from build123d import *

# Parameters (mm, degrees)
SKETCH1_W           = 21
SKETCH1_H           = 15
BOSS_EXTRUDE1_DEPTH = 3
SKETCH2_W           = 4
SKETCH2_H           = 15
BOSS_EXTRUDE2_DEPTH = 14.5
SKETCH3_W           = 4
SKETCH3_H           = 7
SKETCH3_W_2         = 4.5
SKETCH3_H_2         = 4
BOSS_EXTRUDE3_DEPTH = 3.5
FILLET1_R           = 1
FILLET2_R           = 3
FILLET3_R           = 5
SKETCH4_W           = 8
SKETCH4_H           = 10
SKETCH4_R           = 1.75
BOSS_EXTRUDE4_DEPTH = 3
FILLET4_R           = 5
FILLET5_R           = 2
SKETCH7_W           = 8
SKETCH7_H           = 4
BOSS_EXTRUDE5_DEPTH = 10
SKETCH8_W           = 4
SKETCH8_H           = 3
BOSS_EXTRUDE6_DEPTH = 8
SKETCH9_R           = 4.5
CUT_EXTRUDE1_DEPTH  = 5
BOSS_EXTRUDE7_DEPTH = 6.5
SKETCH11_R          = 1.75
SKETCH11_W          = 2
SKETCH11_H          = 7.704965023
BOSS_EXTRUDE8_DEPTH = 3
FILLET6_R           = 4
FILLET7_START       = -17.5
FILLET7_DEPTH       = 3
FILLET7_START_2     = -14.5
FILLET7_2_DEPTH     = 3.464101615
FILLET7_START_3     = -6.795034977
FILLET7_3_DEPTH     = 4.795034977
FILLET8_R           = 3
FILLET9_R           = 3
FILLET10_R          = 1.5


with BuildPart() as part:
    # Sketch1 → Boss-Extrude1 (new body)
    with BuildSketch(Plane.XY):
        Rectangle(SKETCH1_W, SKETCH1_H)
    extrude(amount=-BOSS_EXTRUDE1_DEPTH)

    # Sketch2 → Boss-Extrude2 (add)
    with BuildSketch(Plane(origin=(0, 0, -3), x_dir=(-1, 0, 0), z_dir=(0, 0, -1))):
        with Locations((8.5, 0)):
            Rectangle(SKETCH2_W, SKETCH2_H)
        with Locations((-8.5, 0)):
            Rectangle(SKETCH2_W, SKETCH2_H)
    extrude(amount=BOSS_EXTRUDE2_DEPTH)

    # Sketch3 → Boss-Extrude3 (add)
    with BuildSketch(Plane(origin=(0, 0, -17.5), x_dir=(-1, 0, 0), z_dir=(0, 0, -1))):
        with Locations((8.5, 11)):
            Rectangle(SKETCH3_W, SKETCH3_H)
        with Locations((4.25, 12.5)):
            Rectangle(SKETCH3_W_2, SKETCH3_H_2)
    extrude(amount=-BOSS_EXTRUDE3_DEPTH)

    # Fillet1
    fillet1_edges = [part.edges().sort_by_distance(p)[0] for p in [
        (-6.25, 14.5, -14),
        (-2, 14.5, -15.75),
    ]]
    fillet(fillet1_edges, radius=FILLET1_R)

    # Fillet2
    # the kernel refuses this fillet: 3 mm, written as the material it takes off along each edge
    with BuildSketch(Plane(origin=(-5, 14.5, -17), x_dir=(0, 0, 1), z_dir=(-1, 0, 0))) as fillet2_piece_1:
        with BuildLine():
            CenterArc((2, -1), 1, 0, 90)
            Line((3, -1), (3, 0))
            Line((3, 0), (2, 0))
        make_face()
    revolve(axis=Axis((-5, 14.5, -17), (0, 1, 0)), revolution_arc=90, mode=Mode.SUBTRACT)
    with BuildSketch(Plane(origin=(-2, 14.5, -14), x_dir=(0, 0, -1), z_dir=(0, -1, 0))) as fillet2_piece_2:
        with BuildLine():
            CenterArc((FILLET2_R, -FILLET2_R), FILLET2_R, 90, 90)
            Line((0, -FILLET2_R), (0, 0))
            Line((0, 0), (FILLET2_R, 0))
        make_face()
    extrude(amount=11.5, mode=Mode.SUBTRACT)

    # Fillet3
    # the kernel refuses this fillet: 5 mm, written as the material it adds along each edge
    with BuildSketch(Plane(origin=(-10.5, 7.5, -14), x_dir=(0, 1, 0), z_dir=(1, 0, 0))) as fillet3_piece_1:
        with BuildLine():
            CenterArc((FILLET3_R, FILLET3_R), FILLET3_R, 180, 90)
            Line((0, FILLET3_R), (0, 0))
            Line((0, 0), (FILLET3_R, 0))
        make_face()
    extrude(amount=4)

    # Sketch4 → Boss-Extrude4 (add)
    with BuildSketch(Plane(origin=(0, 0, -17.5), x_dir=(-1, 0, 0), z_dir=(0, 0, -1))):
        with Locations((14.5, 0.098378943)):
            Rectangle(SKETCH4_W, SKETCH4_H)
        with Locations((14.5, 0.098378943)):
            Circle(SKETCH4_R, mode=Mode.SUBTRACT)
    extrude(amount=-BOSS_EXTRUDE4_DEPTH)

    # Fillet4
    # the kernel refuses this fillet: 5 mm, written as the material it adds along each edge
    with BuildSketch(Plane(origin=(-10.5, -4.901621057, -17.5), x_dir=(0, -1, 0), z_dir=(0, 0, 1))) as fillet4_piece_1:
        with BuildLine():
            CenterArc((5, -4.385455085), FILLET4_R, 118.706578905, 61.293421095)
            Line((0, -4.385455085), (0, 0))
            Line((0, 0), (2.598378943, 0))
        make_face()
    extrude(amount=3)
    with BuildSketch(Plane(origin=(-10.5, 5.098378943, -17.5), x_dir=(0, 1, 0), z_dir=(0, 0, 1))) as fillet4_piece_2:
        with BuildLine():
            CenterArc((FILLET4_R, FILLET4_R), FILLET4_R, 180, 90)
            Line((0, FILLET4_R), (0, 0))
            Line((0, 0), (FILLET4_R, 0))
        make_face()
    extrude(amount=3)

    # Fillet5
    fillet5_edges = [part.edges().sort_by_distance(p)[0] for p in [
        (-18.5, 5.098378943, -16),
        (-18.5, -4.901621057, -16),
    ]]
    fillet(fillet5_edges, radius=FILLET5_R)

    # Sketch7 → Boss-Extrude5 (add)
    with BuildSketch(Plane(origin=(10.5, 0, 0), x_dir=(0, 0, -1), z_dir=(1, 0, 0))):
        Polygon((3, -7.5), (0, -7.5), (0, -14.5), (3, -14.5), (3, -10.5), align=None)
        with Locations((7, -12.5)):
            Rectangle(SKETCH7_W, SKETCH7_H)
    extrude(amount=-BOSS_EXTRUDE5_DEPTH)

    # Sketch8 → Boss-Extrude6 (add)
    with BuildSketch(Plane(origin=(0, 0, -3), x_dir=(-1, 0, 0), z_dir=(0, 0, -1))):
        with Locations((-8.5, -9)):
            Rectangle(SKETCH8_W, SKETCH8_H)
    extrude(amount=BOSS_EXTRUDE6_DEPTH)

    # Sketch9 → Cut-Extrude1 (cut)
    with BuildSketch(Plane.XZ.offset(14.5)):
        with Locations((0.5, -11)):
            Circle(SKETCH9_R)
    extrude(amount=-CUT_EXTRUDE1_DEPTH, mode=Mode.SUBTRACT)

    # Sketch10 → Boss-Extrude7 (add)
    with BuildSketch(Plane(origin=(0, 0, -11), x_dir=(-1, 0, 0), z_dir=(0, 0, -1))):
        Polygon((-5, -14.5), (-5, -10.5), (-6.5, -10.5), (-6.5, -7.5), (-10.5, -7.5), (-10.5, -14.5), align=None)
    extrude(amount=BOSS_EXTRUDE7_DEPTH)

    # Sketch11 → Boss-Extrude8 (add)
    # profile 1 of 2: a face of its own
    with BuildSketch(Plane(origin=(0, 0, -17.5), x_dir=(-1, 0, 0), z_dir=(0, 0, -1))):
        Polygon((-5, -23.5), (-5, -14.5), (-10.5, -14.5), (-12.5, -14.5), (-12.5, -23.5), align=None)
        with Locations((-8.75, -19)):
            Circle(SKETCH11_R, mode=Mode.SUBTRACT)
    # profile 2 of 2: a face of its own
    with BuildSketch(Plane(origin=(0, 0, -17.5), x_dir=(-1, 0, 0), z_dir=(0, 0, -1))):
        with Locations((-11.5, -10.647517489)):
            Rectangle(SKETCH11_W, SKETCH11_H)
    extrude(amount=-BOSS_EXTRUDE8_DEPTH)

    # Fillet6
    # the kernel refuses this fillet: 4 mm, written as the material it adds along each edge
    with BuildSketch(Plane(origin=(10.5, -14.5, -14.5), x_dir=(0, 0, 1), z_dir=(0, 1, 0))) as fillet6_piece_1:
        with BuildLine():
            CenterArc((3.464101615, 4), FILLET6_R, 210, 60)
            Line((0, 2), (-0.069282032, 1.96))
            ThreePointArc((-0.069282032, 1.96), (-0.08, 1), (-0.08, 0))
            Line((-0.08, 0), (0, -0.08))
            Line((0, -0.08), (3.464101615, -0.08))
            Line((3.464101615, -0.08), (3.464101615, 0))
        make_face()
    extrude(amount=7.704965023)

    # Fillet7: read off the stored shape, not the designer's step
    # Fillet7 outline → Fillet7 (add)
    with BuildSketch(Plane.XY.offset(FILLET7_START)):
        with BuildLine():
            Line((10.5, -6.795034977), (12.5, -6.795034977))
            ThreePointArc((12.5, -6.795034977), (11.035898385, -5.330933362), (10.5, -3.330933362))
            Line((10.5, -3.330933362), (10.5, -6.795034977))
        make_face()
    extrude(amount=FILLET7_DEPTH)

    # Fillet7 2 outline → Fillet7 2 (add)
    with BuildSketch(Plane.XY.offset(FILLET7_START_2)):
        with BuildLine():
            Line((10.5, -6.795034977), (12.5, -6.795034977))
            ThreePointArc((12.5, -6.795034977), (11.035898385, -5.330933362), (10.5, -3.330933362))
            Line((10.5, -3.330933362), (10.5, -6.795034977))
        make_face()
    extrude(amount=FILLET7_2_DEPTH)

    # Fillet7 3 outline → Fillet7 3 (cut)
    with BuildSketch(Plane(origin=(0, 0, 0), x_dir=(1, 0, 0), z_dir=(0, 1, 0)).offset(FILLET7_START_3)):
        with BuildLine():
            ThreePointArc((12.5, 14.5), (11.035898385, 13.035898385), (10.5, 11.035898385))
            Line((10.5, 11.035898385), (14, 11.035898385))
            Line((14, 11.035898385), (14, 15.366025404))
            Line((14, 15.366025404), (12.5, 14.5))
        make_face()
    extrude(amount=FILLET7_3_DEPTH, mode=Mode.SUBTRACT)

    # Fillet8
    fillet8_edges = [part.edges().sort_by_distance(p)[0] for p in [
        (5, -23.5, -16),
        (12.5, -23.5, -16),
    ]]
    fillet(fillet8_edges, radius=FILLET8_R)

    # Fillet9
    fillet9_edges = [part.edges().sort_by_distance(p)[0] for p in [
        (0.5, -7.5, -1.5),
        (0.5, -12.5, -6.5),
    ]]
    fillet(fillet9_edges, radius=FILLET9_R)

    # Fillet10
    fillet10_edges = [part.edges().sort_by_distance(p)[0] for p in [
        (10.5, -3.5, 0),
        (-10.5, 0, 0),
    ]]
    fillet(fillet10_edges, radius=FILLET10_R)


solid = part.part
CAD build for the part. Positions are in the model's coordinates, mm. A direction names the side the tool comes from. Coordinates: 2 decimals unless noted, no trailing zeros. Write each loop counter-clockwise with the first axis right and the second up, starting at its lowest first coordinate (ties: lowest second). Pieces come first, ordered by that corner, then holes. Notation, with made-up numbers: (-10.5, -6) - (44.5, -6) arc R24 ccw to (44.5, 10) - close; hole circle Ø4 at (80, -15). An arc over 180 degrees is marked (long way). Use a Markdown table: item, result. Add a question column.
Item 1: Mould opens along Y. For faces 6 (the face through (9, -23.5, -16)), 7 (the face through (7, -18, -14.5)), 8 (the face through (8.978, -17.265, -16.021)), 9 (the face through (-7, 14.5, -16)) say: pulls with the +Y half, pulls with the -Y half, needs draft (parallel to the pull), parting line crosses it, or undercut.
Item 2: Band-saw the part on D-D, the plane y = -13. Give the cut face in (x, z), and give its area (3 significant figures).
Item 3: Flat gauge pins, fed straight in: pin 1 (9 mm diameter, centred on x = -8, z = -10, fed in from -Y); pin 2 (4.5 mm diameter, centred on y = -13.5, z = -2.5, fed in from -X); pin 3 (1.5 mm diameter, centred on y = 0.5, z = -15, fed in from +X); pin 4 (8 mm diameter, centred on x = 8, y = 8.5, fed in from -Z). Where does each tip first touch, or does it go through?
Item 4: Band-saw the part on B-B, the plane z = -9.75. Give the cut face in (x, y), and give its area (3 significant figures).
Item 5: Drill centre lines: L1, parallel to X at y = 4, z = -3.25; L2, parallel to Y at x = 8.75, z = -16.4; L3, parallel to Y at x = -14.5, z = -16.05. Where is each one in solid material? Low to high. Write a range as from..to.
Item 6: 3-axis set-ups, long thin cutter, end or side, ignore diameter. For faces 1 (the face through (-16, -4.902, -16)), 2 (the face through (-8.53, 8.93, -12.5)), 3 (the face through (6.5, -2, -10)), 4 (the face through (-12.8, 1.4, -14.5)), 5 (the face through (10.5, -1, -8)): which of +Z, -Z, +X, -X, +Y, -Y reach the whole face in a straight line?
Item 7: Band-saw the part on A-A, the plane y = -19. Give the cut face in (x, z).
Item 8: Band-saw the part on C-C, the plane x = 7.5. Give the cut face in (y, z).
Numbers:
| question | item | result |
|---|---|---|
| 1 | face 6 | pulls with the -Y half |
| 1 | face 7 | needs draft |
| 1 | face 8 | undercut |
| 1 | face 9 | pulls with the +Y half |
| 2 | outline | (0.5, -4.13) arc R3 ccw to (2.3, -6.88) arc R4.5 cw to (5, -11) - (5, -17.5) - (12.5, -17.5) - (12.5, -14.5) arc R4 cw to (10.5, -11.04) - (10.5, -1.5) arc R1.5 ccw to (9, 0) - (0.5, 0) - close |
| 2 | area | 136 mm2 |
| 3 | pin 1 | y = -7.5 |
| 3 | pin 2 | x = 0.5 |
| 3 | pin 3 | x = 10.5 |
| 3 | pin 4 | z = -17.5 |
| 4 | outline | (-10.5, -7.5) - (-6.5, -7.5) - (-6.5, 7.56) - (-10.5, 7.56) - close; (4.82, -14.5) - (10.5, -14.5) - (10.5, 7.5) - (6.5, 7.5) - (6.5, -10.5) - (4.82, -10.5) - close |
| 4 | area | 155 mm2 |
| 5 | L1 | -10.5..-6.5, 6.5..10.5 |
| 5 | L2 | -23.5..-20.75, -17.25..7.5 |
| 5 | L3 | -4.92..-1.65, 1.85..5.2 |
| 6 | face 1 | +Z, -Z, -X, -Y |
| 6 | face 2 | +Z, +X, -X, +Y |
| 6 | face 3 | -Z, +Y |
| 6 | face 4 | +Z, -X, +Y, -Y |
| 6 | face 5 | +Z, +X, +Y |
| 7 | outline | (5, -17.5) - (7, -17.5) - (7, -14.5) - (5, -14.5) - close; (10.5, -17.5) - (12.5, -17.5) - (12.5, -14.5) - (10.5, -14.5) - close |
| 8 | outline | (-23.46, -17.5) - (-20.22, -17.5) - (-20.22, -14.5) - (-23.46, -14.5) - close; (-17.78, -17.5) - (7.5, -17.5) - (7.5, 0) - (-14.5, 0) - (-14.5, -14.5) - (-17.78, -14.5) - close |
